Work out the finished part from the listing and answer in its coordinate system (mm). Round coordinates to 2 decimals unless told otherwise and drop trailing zeros. Write each loop counter-clockwise with the first axis right and the second up, starting at its lowest first coordinate (ties: lowest second). Pieces come first, ordered by that corner, then holes. Notation, with made-up numbers: M -25.5,-28.75 L -14.5,-28.75 A36 ccw -14.5,6.25 Z; hole C 56.5,75.25 d8. An arc over 180 degrees is marked long. Answer in a Markdown table with one row per item.
```python
from build123d import *

# Parameters (mm, degrees)
SKETCH1_R           = 6.25
SKETCH1_R_2         = 1.75
BOSS_EXTRUDE1_DEPTH = 10
SKETCH11_R          = 1.75
CUT_EXTRUDE2_DEPTH  = 10


with BuildPart() as part:
    # Sketch1 → Boss-Extrude1 (new body)
    with BuildSketch(Plane.XY):
        with BuildLine():
            Line((0, 0), (40, 0))
            Line((40, 0), (120, 0))
            Line((120, 0), (160, 0))
            Line((160, 0), (160, 169))
            ThreePointArc((160, 169), (157.656854249, 174.656854249), (152, 177))
            Line((152, 177), (120, 177))
            Line((120, 177), (119.937451095, 177))
            ThreePointArc((119.937451095, 177), (118.319103908, 176.175139303), (118.03566771, 174.380952381))
            ThreePointArc((118.03566771, 174.380952381), (80, 122), (41.96433229, 174.380952381))
            ThreePointArc((41.96433229, 174.380952381), (41.680896092, 176.175139303), (40.062548905, 177))
            Line((40.062548905, 177), (40, 177))
            Line((40, 177), (8, 177))
            ThreePointArc((8, 177), (2.343145751, 174.656854249), (0, 169))
            Line((0, 169), (0, 0))
        make_face()
        with Locations((20, 162)):
            Circle(SKETCH1_R, mode=Mode.SUBTRACT)
        with Locations((140, 162)):
            Circle(SKETCH1_R, mode=Mode.SUBTRACT)
        with Locations((4.328403696, 49)):
            Circle(SKETCH1_R_2, mode=Mode.SUBTRACT)
        with Locations((4.328403696, 29)):
            Circle(SKETCH1_R_2, mode=Mode.SUBTRACT)
        with Locations((36.371302772, 4.5)):
            Circle(SKETCH1_R_2, mode=Mode.SUBTRACT)
        with Locations((123.628697228, 4.5)):
            Circle(SKETCH1_R_2, mode=Mode.SUBTRACT)
        with Locations((155.671596304, 29)):
            Circle(SKETCH1_R_2, mode=Mode.SUBTRACT)
        with Locations((155.671596304, 49)):
            Circle(SKETCH1_R_2, mode=Mode.SUBTRACT)
    extrude(amount=BOSS_EXTRUDE1_DEPTH)

    # Sketch11 → Cut-Extrude2 (cut)
    with BuildSketch(Plane(origin=(0, 0, 0), x_dir=(-1, 0, 0), z_dir=(0, 0, -1))):
        with Locations((-119.515447903, 131.8119911)):
            Circle(SKETCH11_R)
        with Locations((-39.078552479, 133.747183554)):
            Circle(SKETCH11_R)
    extrude(amount=-CUT_EXTRUDE2_DEPTH, mode=Mode.SUBTRACT)


solid = part.part
```
1. The part is cut by section C-C (x = 80). Determine the outline of the cut face in (y, z).
Calculated:
| item | result |
|---|---|
| outline | M 0,0 L 122,0 L 122,10 L 0,10 Z |
2. The part is cut by section A-A (x = 20). Determine the outline of the cut face in (y, z).
Calculated:
| item | result |
|---|---|
| outline | M 0,0 L 155.75,0 L 155.75,10 L 0,10 Z; M 168.25,0 L 177,0 L 177,10 L 168.25,10 Z |
3. Determine the mould class of faces 1 (the flat face through (79, 70, 0)), 2 (the flat face through (0, 86, 5)), 3 (the cylindrical face through (81.056, 122.014, 4.93)), 4 (the flat face through (160, 83, 5)) for opening direction X: released by +X, released by -X, zero draft, split by the parting line, or undercut.
Calculated:
| item | result |
|---|---|
| face 1 | zero draft |
| face 2 | released by -X |
| face 3 | undercut |
| face 4 | released by +X |
4. Consider line 1 along Y through (x, z) = (140, 5); line 2 along Y through (x, z) = (123.5, 2); line 3 along X through (y, z) = (145, 2). Determine where each line is inside the solid, lowest interval first. Write a range as from..to.
Calculated:
| item | result |
|---|---|
| line 1 | y = 0..155.75, 168.25..177 |
| line 2 | y = 0..2.75, 6.25..177 |
| line 3 | x = 0..43.79, 116.21..160 |
5. The part is cut by section B-B (z = 5.25). Count the separate pieces of the cut face and the enclosed holes in it, plus the area to 3 significant figures.
Calculated:
| item | result |
|---|---|
| separate pieces | 1 |
| enclosed holes | 10 |
| area | 24,300 mm² |
6. The part is cut by section D-D (x = 44). Determine the outline of the cut face in (y, z), plus the area to 3 significant figures.
Calculated:
| item | result |
|---|---|
| outline | M 0,0 L 144.56,0 L 144.56,10 L 0,10 Z |
| area | 1,450 mm² |
7. Given pin 1 (3 mm diameter, centred on x = 123.63, y = 4.5, fed in from +Z); pin 2 (5.5 mm diameter, centred on x = 39.08, y = 133.75, fed in from +Z); pin 3 (3 mm diameter, centred on x = 102, z = 7, fed in from +Y); pin 4 (2 mm diameter, centred on x = 55, z = 3.5, fed in from +Y), each flat-ended and moving along its own axis, determine where each tip first touches the part or whether it passes through.
Calculated:
| item | result |
|---|---|
| pin 1 | passes through |
| pin 2 | stops at z = 10 |
| pin 3 | stops at y = 129.63 |
| pin 4 | stops at y = 131.6 |
